CAD build for the part. Positions are in the model's coordinates, mm. Face numbers are marked on the shaded views. A direction names the side the tool comes from. Coordinates: 2 decimals unless noted, no trailing zeros. Loops run counter-clockwise (first coordinate to the right, second up) from the corner with the lowest first, then second, coordinate; pieces in that order, holes last. Notation, with made-up numbers: (0, -14.5) -> (42, -14.5) arc R35 cw to (42, 20.5) -> close; hole circle Ø5 at (-37, -39). An arc over 180 degrees is marked (long way). Write each question's results on one line, items separated by ' | '.
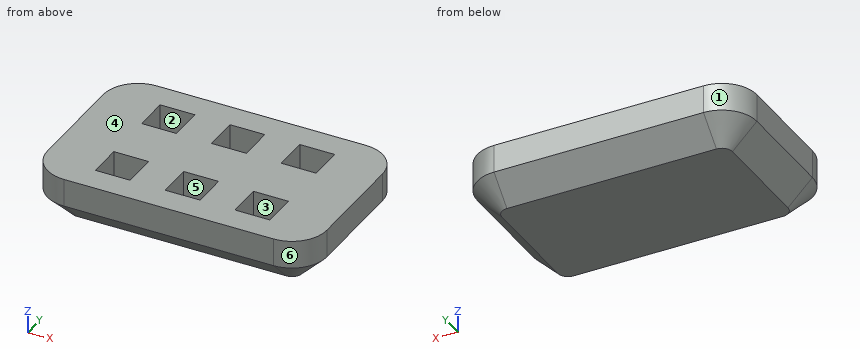
from build123d import *

# Parameters (mm, degrees)
F0_W     = 12.7
F0_H     = 12.7
F1_DEPTH = 38.1
F2_DEPTH = 25.4
F3_R     = 25.4
F4_SIZE  = 17.78


with BuildPart() as f1:
    # F0 (on Top) → F1 (new body)
    with BuildSketch(Plane.XY):
        Polygon((101.6, 63.5), (-101.6, 63.5), (-101.6, 31.75), (-63.5, 31.75), (-63.5, 44.45), (-38.1, 44.45), (-38.1, 31.75), (-12.7, 31.75), (-12.7, 44.45), (12.7, 44.45), (12.7, 31.75), (38.1, 31.75), (38.1, 44.45), (63.5, 44.45), (63.5, 31.75), (101.6, 31.75), align=None)
        Polygon((-63.5, 31.75), (-101.6, 31.75), (-101.6, -31.75), (-63.5, -31.75), (-63.5, -19.05), (-38.1, -19.05), (-38.1, -31.75), (-12.7, -31.75), (-12.7, -19.05), (0, -19.05), (0, 0), (0, 19.05), (-12.7, 19.05), (-12.7, 31.75), (-38.1, 31.75), (-38.1, 19.05), (-63.5, 19.05), align=None)
        Polygon((101.6, -31.75), (101.6, 31.75), (63.5, 31.75), (63.5, 19.05), (38.1, 19.05), (38.1, 31.75), (12.7, 31.75), (12.7, 19.05), (0, 19.05), (0, 0), (0, -19.05), (12.7, -19.05), (12.7, -31.75), (38.1, -31.75), (38.1, -19.05), (63.5, -19.05), (63.5, -31.75), align=None)
        Polygon((-63.5, -31.75), (-101.6, -31.75), (-101.6, -63.5), (101.6, -63.5), (101.6, -31.75), (63.5, -31.75), (63.5, -44.45), (38.1, -44.45), (38.1, -31.75), (12.7, -31.75), (12.7, -44.45), (-12.7, -44.45), (-12.7, -31.75), (-38.1, -31.75), (-38.1, -44.45), (-63.5, -44.45), align=None)
        Polygon((-50.8, 31.75), (-63.5, 31.75), (-63.5, 19.05), (-38.1, 19.05), (-38.1, 31.75), align=None)
        Polygon((-63.5, 44.45), (-63.5, 31.75), (-50.8, 31.75), (-38.1, 31.75), (-38.1, 44.45), align=None)
        Polygon((-12.7, 44.45), (-12.7, 31.75), (0, 31.75), (12.7, 31.75), (12.7, 44.45), align=None)
        with Locations((-6.35, 25.4)):
            Rectangle(F0_W, F0_H)
        with Locations((6.35, 25.4)):
            Rectangle(F0_W, F0_H)
        Polygon((63.5, 19.05), (63.5, 31.75), (50.8, 31.75), (38.1, 31.75), (38.1, 19.05), align=None)
        Polygon((50.8, 31.75), (63.5, 31.75), (63.5, 44.45), (38.1, 44.45), (38.1, 31.75), align=None)
        Polygon((50.8, -31.75), (63.5, -31.75), (63.5, -19.05), (38.1, -19.05), (38.1, -31.75), align=None)
        Polygon((63.5, -44.45), (63.5, -31.75), (50.8, -31.75), (38.1, -31.75), (38.1, -44.45), align=None)
        Polygon((0, -31.75), (-12.7, -31.75), (-12.7, -44.45), (12.7, -44.45), (12.7, -31.75), align=None)
        with Locations((-6.35, -25.4)):
            Rectangle(F0_W, F0_H)
        with Locations((6.35, -25.4)):
            Rectangle(F0_W, F0_H)
        Polygon((-63.5, -19.05), (-63.5, -31.75), (-50.8, -31.75), (-38.1, -31.75), (-38.1, -19.05), align=None)
        Polygon((-50.8, -31.75), (-63.5, -31.75), (-63.5, -44.45), (-38.1, -44.45), (-38.1, -31.75), align=None)
    extrude(amount=-F1_DEPTH)

    # F0 (on Top) → F2 (cut)
    with BuildSketch(Plane.XY):
        Polygon((-63.5, 44.45), (-63.5, 31.75), (-50.8, 31.75), (-38.1, 31.75), (-38.1, 44.45), align=None)
        Polygon((-50.8, 31.75), (-63.5, 31.75), (-63.5, 19.05), (-38.1, 19.05), (-38.1, 31.75), align=None)
        Polygon((-63.5, -19.05), (-63.5, -31.75), (-50.8, -31.75), (-38.1, -31.75), (-38.1, -19.05), align=None)
        Polygon((-50.8, -31.75), (-63.5, -31.75), (-63.5, -44.45), (-38.1, -44.45), (-38.1, -31.75), align=None)
        with Locations((-6.35, -25.4)):
            Rectangle(F0_W, F0_H)
        with Locations((6.35, -25.4)):
            Rectangle(F0_W, F0_H)
        with Locations((-6.35, 25.4)):
            Rectangle(F0_W, F0_H)
        with Locations((6.35, 25.4)):
            Rectangle(F0_W, F0_H)
        Polygon((-12.7, 44.45), (-12.7, 31.75), (0, 31.75), (12.7, 31.75), (12.7, 44.45), align=None)
        Polygon((0, -31.75), (-12.7, -31.75), (-12.7, -44.45), (12.7, -44.45), (12.7, -31.75), align=None)
        Polygon((63.5, -44.45), (63.5, -31.75), (50.8, -31.75), (38.1, -31.75), (38.1, -44.45), align=None)
        Polygon((50.8, -31.75), (63.5, -31.75), (63.5, -19.05), (38.1, -19.05), (38.1, -31.75), align=None)
        Polygon((63.5, 19.05), (63.5, 31.75), (50.8, 31.75), (38.1, 31.75), (38.1, 19.05), align=None)
        Polygon((50.8, 31.75), (63.5, 31.75), (63.5, 44.45), (38.1, 44.45), (38.1, 31.75), align=None)
    extrude(amount=-F2_DEPTH, mode=Mode.SUBTRACT)

    # F3
    f3_edges = [f1.edges().sort_by_distance(p)[0] for p in [
        (-101.6, -63.5, -19.05),
        (101.6, -63.5, -19.05),
        (101.6, 63.5, -19.05),
        (-101.6, 63.5, -19.05),
    ]]
    fillet(f3_edges, radius=F3_R)

    # F4
    f4_edges = [f1.edges().sort_by_distance(p)[0] for p in [
        (0, -63.5, -38.1),
    ]]
    chamfer(f4_edges, length=F4_SIZE)


solid = f1.part
1) Slice it at A-A (z = -15). Count the separate pieces of the cut face and the enclosed holes in it, then the cut area to 3 significant figures.
Outcome:
separate pieces: 1 | enclosed holes: 6 | area: 21,400 mm^2
2) Slice it at B-B (y = 33). Write the cut outline in (x, z), then the cut area to 3 significant figures.
Outcome:
outline: (-101.6, -20.32) -> (-83.82, -38.1) -> (83.82, -38.1) -> (101.6, -20.32) -> (101.6, 0) -> (63.5, 0) -> (63.5, -25.4) -> (38.1, -25.4) -> (38.1, 0) -> (12.7, 0) -> (12.7, -25.4) -> (-12.7, -25.4) -> (-12.7, 0) -> (-38.1, 0) -> (-38.1, -25.4) -> (-63.5, -25.4) -> (-63.5, 0) -> (-101.6, 0) -> close | area: 5,490 mm^2
3) Slice it at C-C (x = -49.5). Write the cut outline in (y, z), then the cut area to 3 significant figures.
Outcome:
outline: (-63.5, -20.32) -> (-45.72, -38.1) -> (45.72, -38.1) -> (63.5, -20.32) -> (63.5, 0) -> (44.45, 0) -> (44.45, -25.4) -> (19.05, -25.4) -> (19.05, 0) -> (-19.05, 0) -> (-19.05, -25.4) -> (-44.45, -25.4) -> (-44.45, 0) -> (-63.5, 0) -> close | area: 3,230 mm^2
4) Drill centre lines: L1, parallel to X at y = 38.5, z = -15; L2, parallel to Y at x = 54, z = -17; L3, parallel to X at y = -44, z = -2.5. Where is each one in solid material? Low to high. Write a range as from..to.
Outcome:
L1: x = -101.6..-63.5, -38.1..-12.7, 12.7..38.1, 63.5..101.6 | L2: y = -63.5..-44.45, -19.05..19.05, 44.45..63.5 | L3: x = -100.91..-63.5, -38.1..-12.7, 12.7..38.1, 63.5..100.91
5) Slice it at D-D (z = -35). Write the cut outline in (x, y), then the cut area to 3 significant figures.
Outcome:
outline: (-86.92, -38.1) arc R10.72 ccw to (-76.2, -48.82) -> (76.2, -48.82) arc R10.72 ccw to (86.92, -38.1) -> (86.92, 38.1) arc R10.72 ccw to (76.2, 48.82) -> (-76.2, 48.82) arc R10.72 ccw to (-86.92, 38.1) -> close | area: 16,900 mm^2
6) Pin check, flat tips, straight feed: pin 1 (7.5 mm diameter, centred on x = 55.5, y = -26.5, fed in from +Z); pin 2 (4 mm diameter, centred on x = 41, y = 48.5, fed in from -Z); pin 3 (10 mm diameter, centred on x = -53, y = -11, fed in from +Z); pin 4 (1.5 mm diameter, centred on x = 79.5, z = -6.5, fed in from +Y). Stop position of each tip, or through.
Outcome:
pin 1: stops at z = -25.4 | pin 2: stops at z = -37.32 | pin 3: stops at z = 0 | pin 4: stops at y = 63.37
7) Which spindle directions (+Z, -Z, +X, -X, +Y, -Y) get a long thin tool onto all of the face, cutting with end or side? Do the marked faces 5 and 6. Say none if no direction does.
Outcome:
face 5: +Z | face 6: +Z, -Z, +X, -Y
8) Two-plate mould, pull along X, no slides. Class the marked faces 1, 2, 3 and 4: pulls with the +X half, pulls with the -X half, needs draft (parallel to the pull), parting line crosses it, or undercut.
Outcome:
face 1: pulls with the -X half | face 2: undercut | face 3: undercut | face 4: needs draft
